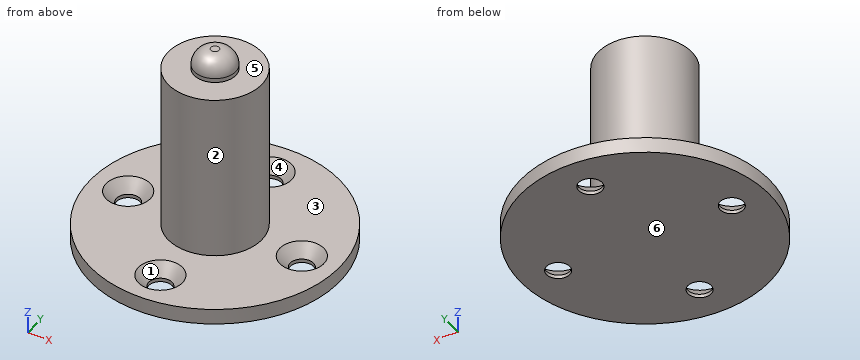
from build123d import *

# Parameters (mm, degrees)
F0_R            = 38.1
F1_DEPTH        = 4.7625
F2_R            = 14.2875
F3_DEPTH        = 50.8
F4_R            = 6.35
F5_DEPTH        = 6.35
F6_R            = 5.08
F8_D            = 7.1374
F8_DEPTH        = 15.875
F8_CSINK_D      = 13.4874
F8_CSINK_ANGLE  = 82
F8_TIP          = 2.1442912911
F8_COPIES_COUNT = 4


# Not quite as in the source:
# - a pattern or mirror of a feature is missing from the dataset's text; its kind, count and spacing are read off the source's solid


with BuildPart() as f1:
    # F0 (on Top) → F1 (new body)
    with BuildSketch(Plane.XY):
        Circle(F0_R)
    extrude(amount=F1_DEPTH)

    # F2 (on face) → F3 (join)
    with BuildSketch(Plane.XY.offset(4.7625)):
        Circle(F2_R)
    extrude(amount=F3_DEPTH)

    # F4 (on face) → F5 (join)
    with BuildSketch(Plane.XY.offset(55.5625)):
        Circle(F4_R)
    extrude(amount=F5_DEPTH)

    # F6
    f6_edges = [f1.edges().sort_by_distance(p)[0] for p in [
        (-6.35, 0, 61.9125),
    ]]
    fillet(f6_edges, radius=F6_R)

    # F8
    with Locations(Plane.XY.offset(4.7625)):
        with Locations((0, -26.9875)):
            f8 = CounterSinkHole(F8_D / 2, F8_CSINK_D / 2, depth=F8_DEPTH, counter_sink_angle=F8_CSINK_ANGLE)
            with Locations((0, 0, -(F8_DEPTH + F8_TIP / 2))):  # 118° drill point
                Cone(0, F8_D / 2, F8_TIP, mode=Mode.SUBTRACT)

    # F8_copies: F8 ×4 about axis
    f8_copies_axis = Axis((0, 0, 0), (0, 0, 1))
    for i in range(1, F8_COPIES_COUNT):
        add(f8.rotate(f8_copies_axis, i * 360 / F8_COPIES_COUNT), mode=Mode.SUBTRACT)


solid = f1.part
Input: part model. Units: mm. Frame: model coordinates. Face numbers are marked on the shaded views. A direction names the side the tool comes from. Coordinates: 2 decimals unless noted, no trailing zeros. Loops run counter-clockwise (first coordinate to the right, second up) from the corner with the lowest first, then second, coordinate; pieces in that order, holes last.
(1) Section C-C on z = 46.5. Return the cut outline in (x, y) (1 decimal), then the cut area to 3 significant figures.
(2) Set-up query: the marked faces 5 and 6. Return all of +Z, -Z, +X, -X, +Y, -Y with unobstructed straight access to the full face (end or side cutting, diameter ignored); none if empty.
(3) First-contact query: pin 1 Ø4 at (y, z) = (15, 8) entering from +X; pin 2 Ø2 at (x, y) = (-9, -9) entering from +Z; pin 3 Ø8 at (x, y) = (0, 26.99) entering from +Z. Flat tips, straight axial feed; report the tip coordinate or a pass-through.
(4) Pull-direction query (X, two-part tool) for the marked faces 1, 2, 3 and 4; classes: released by +X, released by -X, zero draft, split by the parting line, or undercut.
(5) Section D-D on x = 11.5. Return the cut outline in (y, z), then the cut area to 3 significant figures.
(6) Material intervals for probe 1 along Y at (x, z) = (0, 0.75); probe 2 along Z at (x, y) = (-12, -22); probe 3 along Z at (x, y) = (-4, 8.5), sorted ascending.
(7) Section A-A on y = 0. Count the separate pieces of the cut face and the enclosed holes in it, then the cut area to 3 significant figures.
Data:
1. outline: circle Ø28.6 at (0, 0)
1. area: 641 mm2
2. face 5: +Z
2. face 6: -Z, +X, -X, +Y, -Y
3. pin 1: stops at x = 5.93
3. pin 2: stops at z = 55.56
3. pin 3: stops at z = 1.61
4. face 1: undercut
4. face 2: split by the parting line
4. face 3: zero draft
4. face 4: undercut
5. outline: (-36.32, 0) - (36.32, 0) - (36.32, 4.76) - (8.48, 4.76) - (8.48, 55.56) - (-8.48, 55.56) - (-8.48, 4.76) - (-36.32, 4.76) - close
5. area: 1,210 mm2
6. probe 1: y = -38.1 to -30.56, -23.42 to 23.42, 30.56 to 38.1
6. probe 2: z = 0 to 4.76
6. probe 3: z = 0 to 55.56
7. separate pieces: 3
7. enclosed holes: 0
7. area: 1,790 mm2
